```python
from build123d import *

# Parameters (mm, degrees)
BOSS_EXTRUDE1_DEPTH = 12.7
CUT_EXTRUDE1_DEPTH  = 25.379038558
CUT_EXTRUDE2_DEPTH  = 2.6035
CUT_EXTRUDE3_DEPTH  = 23.735837812
CUT_EXTRUDE4_DEPTH  = 4.318


with BuildPart() as part:
    # Sketch1 → Boss-Extrude1 (new body)
    with BuildSketch(Plane(origin=(0, 0, 0), x_dir=(1, 0, 0), z_dir=(0, 1, 0))):
        with BuildLine():
            Line((-15.621, -5.08), (15.621, -5.08))
            ThreePointArc((15.621, -5.08), (17.417051224, -4.336051224), (18.161, -2.54))
            Line((18.161, -2.54), (18.161, 2.54))
            ThreePointArc((18.161, 2.54), (17.417051224, 4.336051224), (15.621, 5.08))
            Line((15.621, 5.08), (-15.621, 5.08))
            ThreePointArc((-15.621, 5.08), (-17.417051224, 4.336051224), (-18.161, 2.54))
            Line((-18.161, 2.54), (-18.161, -2.54))
            ThreePointArc((-18.161, -2.54), (-17.417051224, -4.336051224), (-15.621, -5.08))
        make_face()
    extrude(amount=BOSS_EXTRUDE1_DEPTH)

    # Sketch2 → Cut-Extrude1 (cut, through all)
    with BuildSketch(Plane.XY.offset(5.08)):
        with BuildLine():
            Line((-6.35, 0), (6.35, 0))
            ThreePointArc((6.35, 0), (0, 6.35), (-6.35, 0))
        make_face()
    extrude(amount=-CUT_EXTRUDE1_DEPTH, mode=Mode.SUBTRACT)

    # Sketch3 → Cut-Extrude2 (cut, symmetric)
    with BuildSketch(Plane.XY):
        with BuildLine():
            Line((-8.001, 0), (8.001, 0))
            ThreePointArc((8.001, 0), (0, 8.001), (-8.001, 0))
        make_face()
    extrude(amount=CUT_EXTRUDE2_DEPTH, both=True, mode=Mode.SUBTRACT)

    # Sketch4 → Cut-Extrude3 (cut, through all)
    with BuildSketch(Plane.XZ):
        with BuildLine():
            Line((12.065, 2.286), (13.335, 2.286))
            ThreePointArc((13.335, 2.286), (15.621, 0), (13.335, -2.286))
            Line((13.335, -2.286), (12.065, -2.286))
            ThreePointArc((12.065, -2.286), (9.779, 0), (12.065, 2.286))
        make_face()
        with BuildLine():
            Line((-13.335, 2.286), (-12.065, 2.286))
            ThreePointArc((-12.065, 2.286), (-9.779, 0), (-12.065, -2.286))
            Line((-12.065, -2.286), (-13.335, -2.286))
            ThreePointArc((-13.335, -2.286), (-15.621, 0), (-13.335, 2.286))
        make_face()
    extrude(amount=-CUT_EXTRUDE3_DEPTH, mode=Mode.SUBTRACT)

    # Sketch5 → Cut-Extrude4 (cut)
    with BuildSketch(Plane(origin=(0, 12.7, 0), x_dir=(1, 0, 0), z_dir=(0, 1, 0))):
        with BuildLine():
            Line((-12.065, 3.81), (-13.335, 3.81))
            ThreePointArc((-13.335, 3.81), (-17.145, 0), (-13.335, -3.81))
            Line((-13.335, -3.81), (-12.065, -3.81))
            ThreePointArc((-12.065, -3.81), (-8.255, 0), (-12.065, 3.81))
        make_face()
        with BuildLine():
            Line((12.065, -3.556), (13.335, -3.556))
            ThreePointArc((13.335, -3.556), (16.891, 0), (13.335, 3.556))
            Line((13.335, 3.556), (12.065, 3.556))
            ThreePointArc((12.065, 3.556), (8.509, 0), (12.065, -3.556))
        make_face()
    extrude(amount=-CUT_EXTRUDE4_DEPTH, mode=Mode.SUBTRACT)


solid = part.part
```
Work out the finished part from the listing and answer in its coordinate system (mm). A direction names the side the tool comes from. Give positions to 0.01 mm unless a question says otherwise; leave off trailing zeros. Loops run counter-clockwise (first coordinate to the right, second up) from the corner with the lowest first, then second, coordinate; pieces in that order, holes last. Notation, with made-up numbers: (25, -37) -> (61, -37) arc R28 ccw to (61, -17) -> close; hole circle Ø9 at (4, -33.75). An arc over 180 degrees is marked (long way). Write item = value, one per line. Start each with the question number.
(1) Find the intervals of material crossed by probe 1 along Z at (x, y) = (-4.5, 5.75); probe 2 along X at (y, z) = (11.75, -2.75); probe 3 along X at (y, z) = (12.25, 3), in increasing order. Write a range as from..to.
(2) The mould has two halves that part along X. Classify faces 4 (the flat face through (-18.161, 6, 0)), 5 (the cylindrical face through (-15.62, 4.13, -0.05)), 6 (the flat face through (10.9, 0, -2.3)): +X half, -X half, draft (parallel to the pull), parting line (faces both ways), or undercut.
(3) Find section A-A on y = 2. Give the vertices of the cut face in (x, z) (1 decimal).
(4) Find section C-C on x = -11. Give the vertices of the cut face in (y, z), and give its area (3 significant figures).
(5) Given pin 1 Ø1.5 at (x, z) = (-5, 2.5) entering from -Y; pin 2 Ø4 at (x, y) = (2, 3.5) entering from +Z; pin 3 Ø1.5 at (y, z) = (10, -3) entering from +X; pin 4 Ø3.5 at (x, z) = (14.5, 0.5) entering from +Y, each flat-ended and moving along its own axis, determine where each tip first touches the part or whether it passes through.
(6) Which of the six approach directions +Z, -Z, +X, -X, +Y, -Y give full straight-line access (tool end or side, diameter ignored) to faces 1 (the cylindrical face through (0, 8, 0)), 2 (the flat face through (13, 11, -3.556)), 3 (the flat face through (13, 4, -2.286))?
(7) Find section D-D on x = 0. Give the vertices of the cut face in (y, z).
(8) Find section B-B on z = 0. Give the vertices of the cut face in (x, y) (3 decimals).
From the geometry:
q1.probe_1 = -5.08..-2.6, 2.6..5.08
q1.probe_2 = -18.15..-15.97, -9.43..9.81, 15.59..18.15
q1.probe_3 = -18.12..-15.68, -9.72..10.16, 15.24..18.12
q2.face_4 = -X half
q2.face_5 = undercut
q2.face_6 = draft
q3.outline = (-18.2, -2.5) arc R2.5 ccw to (-15.6, -5.1) -> (-6, -5.1) -> (-6, -2.6) -> (-7.7, -2.6) -> (-7.7, 2.6) -> (-6, 2.6) -> (-6, 5.1) -> (-15.6, 5.1) arc R2.5 ccw to (-18.2, 2.5) -> close; (6, -5.1) -> (15.6, -5.1) arc R2.5 ccw to (18.2, -2.5) -> (18.2, 2.5) arc R2.5 ccw to (15.6, 5.1) -> (6, 5.1) -> (6, 2.6) -> (7.7, 2.6) -> (7.7, -2.6) -> (6, -2.6) -> close; hole (-13.3, -2.3) -> (-12.1, -2.3) arc R2.3 ccw to (-12.1, 2.3) -> (-13.3, 2.3) arc R2.3 ccw to start; hole (12.1, -2.3) -> (13.3, -2.3) arc R2.3 ccw to (13.3, 2.3) -> (12.1, 2.3) arc R2.3 ccw to start
q4.outline = (0, -5.08) -> (12.7, -5.08) -> (12.7, -3.66) -> (8.38, -3.66) -> (8.38, -2.02) -> (0, -2.02) -> close; (0, 2.02) -> (8.38, 2.02) -> (8.38, 3.66) -> (12.7, 3.66) -> (12.7, 5.08) -> (0, 5.08) -> close
q4.area = 63.5 mm^2
q5.pin_1 = 2.71
q5.pin_2 = through
q5.pin_3 = 18.16
q5.pin_4 = 8.38
q6.face_1 = -Y
q6.face_2 = +Y
q6.face_3 = +Y, -Y
q7.outline = (6.35, -5.08) -> (12.7, -5.08) -> (12.7, 5.08) -> (6.35, 5.08) -> (6.35, 2.6) -> (8, 2.6) -> (8, -2.6) -> (6.35, -2.6) -> close
q8.outline = (-18.161, 0) -> (-15.621, 0) -> (-15.621, 8.382) -> (-17.145, 8.382) -> (-17.145, 12.7) -> (-18.161, 12.7) -> close; (-9.779, 0) -> (-8.001, 0) arc R8.001 cw to (8.001, 0) -> (9.779, 0) -> (9.779, 8.382) -> (8.509, 8.382) -> (8.509, 12.7) -> (-8.255, 12.7) -> (-8.255, 8.382) -> (-9.779, 8.382) -> close; (15.621, 0) -> (18.161, 0) -> (18.161, 12.7) -> (16.891, 12.7) -> (16.891, 8.382) -> (15.621, 8.382) -> close
